Design review of the part built by this model. Coordinates are the model's own, in mm. A direction names the side the tool comes from. Round coordinates to 2 decimals unless told otherwise and drop trailing zeros. Order: outer loops, then holes, each group sorted by start corner. A loop starts at its lowest first (then second) coordinate and runs counter-clockwise, first axis right, second up. Notation, with made-up numbers: (29.5, 87) - (52.5, 87) arc R19 cw to (52.5, 109) - close; hole circle Ø4 at (38.25, -11). An arc over 180 degrees is marked (long way). Answer as a JSON object with one key per item and string values. Group by question number.
from build123d import *

# Parameters (mm, degrees)
F0_W     = 127
F0_H     = 127
F1_DEPTH = 635
F2_R     = 38.1
F3_DEPTH = 127.001
F5_DEPTH = 635.001


with BuildPart() as f1:
    # F0 (on Front) → F1 (new body)
    with BuildSketch(Plane.XZ):
        Rectangle(F0_W, F0_H)
    extrude(amount=F1_DEPTH)

    # F2 (on face) → F3 (cut, through all)
    with BuildSketch(Plane.XY.offset(63.5)):
        with Locations((0, -360.032264)):
            Circle(F2_R)
    extrude(amount=-F3_DEPTH, mode=Mode.SUBTRACT)

    # F4 (on face) → F5 (cut, through all)
    with BuildSketch(Plane.XZ.offset(635)):
        Polygon((19.05, -32.995568), (38.1, 0), (19.05, 32.995568), (-19.05, 32.995568), (-38.1, 0), (-19.05, -32.995568), align=None)
    extrude(amount=-F5_DEPTH, mode=Mode.SUBTRACT)


solid = f1.part
1. Take a section at B-B, the plane y = -590. Give the boundary of the cut face in (x, z).
2. Take a section at D-D, the plane y = -387. Give the boundary of the cut face in (x, z), then the cut area to 3 significant figures.
3. Take a section at C-C, the plane z = -51.5. Give the boundary of the cut face in (x, y).
4. Take a section at A-A, the plane x = 0. Give the boundary of the cut face in (y, z).
5. Mouldability with a two-part tool opening along Z and no side actions: class faces 1 (the flat face through (28.44, -182.54, -16.73)), 2 (the flat face through (-1, -313, 63.5)), 3 (the flat face through (27, -635, 29)) as pulls with the +Z half, pulls with the -Z half, needs draft (parallel to the pull), parting line crosses it, or undercut.
6. Tool access review of faces 4 (the flat face through (63.5, -313, -1)), 5 (the flat face through (-28.708, -182.536, -16.267)): name each direction out of +Z, -Z, +X, -X, +Y, -Y from which nothing blocks a thin tool from reaching the whole face with its end or side.
7. To check wall thickness, follow line 1 (Z direction, x = 7, y = -64); line 2 (Y direction, x = -1.5, z = 51); line 3 (Y direction, x = 0, z = 46). State the ranges of each line that lie inside material, in increasing order. Write a range as from..to.
8. Clearance check with a flat-ended pin moving along its axis: P1, Ø2, axis at x = -44.5, z = -50, coming from the +Y side. State where the tip first meets the part, or that it passes through.
Response values:
{
 "1": {"outline": "(-63.5, -63.5) - (63.5, -63.5) - (63.5, 63.5) - (-63.5, 63.5) - close; hole (-38.1, 0) - (-19.05, -33) - (19.05, -33) - (38.1, 0) - (19.05, 33) - (-19.05, 33) - close"},
 "2": {"outline": "(-63.5, -63.5) - (-26.91, -63.5) - (-26.91, -19.38) - (-38.1, 0) - (-26.91, 19.38) - (-26.91, 63.5) - (-63.5, 63.5) - close; (26.91, -63.5) - (63.5, -63.5) - (63.5, 63.5) - (26.91, 63.5) - (26.91, 19.38) - (38.1, 0) - (26.91, -19.38) - close", "area": "8,860 mm2"},
 "3": {"outline": "(-63.5, -635) - (63.5, -635) - (63.5, 0) - (-63.5, 0) - close; hole circle Ø76.2 at (0, -360.03)"},
 "4": {"outline": "(-635, -63.5) - (-398.13, -63.5) - (-398.13, -33) - (-635, -33) - close; (-635, 33) - (-398.13, 33) - (-398.13, 63.5) - (-635, 63.5) - close; (-321.93, -63.5) - (0, -63.5) - (0, -33) - (-321.93, -33) - close; (-321.93, 33) - (0, 33) - (0, 63.5) - (-321.93, 63.5) - close"},
 "5": {"face 1": "undercut", "face 2": "pulls with the +Z half", "face 3": "needs draft"},
 "6": {"face 4": "+Z, -Z, +X, +Y, -Y", "face 5": "+Y, -Y"},
 "7": {"line 1": "-63.5..-33, 33..63.5", "line 2": "-635..-398.1, -321.96..0", "line 3": "-635..-398.13, -321.93..0"},
 "8": {"P1": "y = 0"}
}
